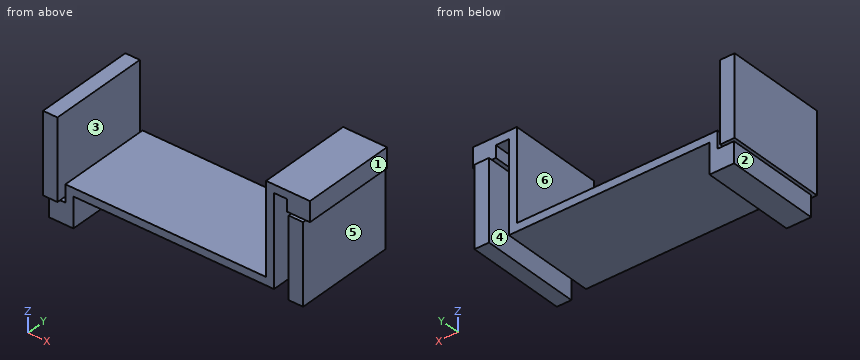
```python
from build123d import *

# Parameters (mm, degrees)
MALE_START                                 = 10.1
SKETCH_1_W                                 = 2.54
SKETCH_1_H                                 = 17.78
MALE_HOUSINGS_IN_J5_DEPTH                  = 14
FEMALE_START                               = 8.66
SKETCH_2_W                                 = 2.54
SKETCH_2_H                                 = 17.78
FEMALE_HOUSINGS_ON_THE_MODULE_HEADER_DEPTH = 14
S_BEND_START                               = 5
SKETCH_3_W                                 = 4.3
SKETCH_3_H                                 = 16.64
S_BEND_ABOVE_THE_FEMALE_HOUSINGS_DEPTH     = 3.66
SKETCH_4_W                                 = 1.4
SKETCH_4_H                                 = 16.64
S_BEND_DOWN_LEG_DEPTH                      = 6.7
RUN_START                                  = 10.3
SKETCH_5_W                                 = 36.6
SKETCH_5_H                                 = 16.64
RUN_UNDER_THE_BATTERY_DEPTH                = 1.4
DROP_START                                 = 10.3
SKETCH_6_W                                 = 1.4
SKETCH_6_H                                 = 16.64
DROP_BESIDE_THE_MODULE_EDGE_DEPTH          = 17.3
RUN_START_2                                = 26.2
SKETCH_7_W                                 = 7.7
SKETCH_7_H                                 = 16.64
RUN_UNDER_THE_MALE_HOUSINGS_DEPTH          = 1.4
LOOP_START                                 = 24.1
SKETCH_8_W                                 = 4
SKETCH_8_H                                 = 16.64
LOOP_INTO_THE_MALE_HOUSINGS_DEPTH          = 3.5


with BuildPart() as part:
    # 草圖1 → male housings in J5 (new body)
    with BuildSketch(Plane.XY.offset(MALE_START)):
        with Locations((56, 45)):
            Rectangle(SKETCH_1_W, SKETCH_1_H)
    extrude(amount=MALE_HOUSINGS_IN_J5_DEPTH)



with BuildPart() as body_2:
    # 草圖2 → female housings on the module header (new body)
    with BuildSketch(Plane.XY.offset(FEMALE_START)):
        with Locations((12.9, 45)):
            Rectangle(SKETCH_2_W, SKETCH_2_H)
    extrude(amount=FEMALE_HOUSINGS_ON_THE_MODULE_HEADER_DEPTH)

    # 草圖3 → S-bend above the female housings (add)
    with BuildSketch(Plane.XY.offset(S_BEND_START)):
        with Locations((14.35, 45)):
            Rectangle(SKETCH_3_W, SKETCH_3_H)
    extrude(amount=S_BEND_ABOVE_THE_FEMALE_HOUSINGS_DEPTH)

    # 草圖4 → S-bend down leg (add)
    with BuildSketch(Plane.XY.offset(S_BEND_START)):
        with Locations((15.8, 45)):
            Rectangle(SKETCH_4_W, SKETCH_4_H)
    extrude(amount=S_BEND_DOWN_LEG_DEPTH)

    # 草圖5 → run under the battery (add)
    with BuildSketch(Plane.XY.offset(RUN_START)):
        with Locations((33.4, 45)):
            Rectangle(SKETCH_5_W, SKETCH_5_H)
    extrude(amount=RUN_UNDER_THE_BATTERY_DEPTH)

    # 草圖6 → drop beside the module edge (add)
    with BuildSketch(Plane.XY.offset(DROP_START)):
        with Locations((51, 45)):
            Rectangle(SKETCH_6_W, SKETCH_6_H)
    extrude(amount=DROP_BESIDE_THE_MODULE_EDGE_DEPTH)

    # 草圖7 → run under the male housings (add)
    with BuildSketch(Plane.XY.offset(RUN_START_2)):
        with Locations((54.15, 45)):
            Rectangle(SKETCH_7_W, SKETCH_7_H)
    extrude(amount=RUN_UNDER_THE_MALE_HOUSINGS_DEPTH)


with BuildPart() as part_1:
    add(part.part)

    add(body_2.part)  # loop into the male housings merges body 2
    # 草圖8 → loop into the male housings (add)
    with BuildSketch(Plane.XY.offset(LOOP_START)):
        with Locations((56, 45)):
            Rectangle(SKETCH_8_W, SKETCH_8_H)
    extrude(amount=LOOP_INTO_THE_MALE_HOUSINGS_DEPTH)


solid = part_1.part
```
Read the model definition and answer for the solid it produces. Units are mm, in the model's axes. Face numbers are marked on the shaded views. A direction names the side the tool comes from. Give positions to 0.01 mm unless a question says otherwise; leave off trailing zeros. Order: outer loops, then holes, each group sorted by start corner. A loop starts at its lowest first (then second) coordinate and runs counter-clockwise, first axis right, second up.
(1) Find section B-B (y = 52.5). Give the vertices of the cut face in (x, z).
(2) Find section D-D (x = 51). Give the vertices of the cut face in (y, z), plus the area to 3 significant figures.
(3) Find section A-A (z = 19.25). Give the vertices of the cut face in (x, y).
(4) For a pull along X with two mould halves and no side action, classify the marked faces 1, 2 and 3 as released by +X, released by -X, zero draft, split by the parting line, or undercut.
(5) Given pin 1 (8 mm diameter, centred on x = 51, y = 52, fed in from -Z); pin 2 (2 mm diameter, centred on x = 13, y = 49, fed in from +Z); pin 3 (8.5 mm diameter, centred on x = 37.5, y = 42, fed in from +Z); pin 4 (0.6 mm diameter, centred on x = 55.5, y = 36.5, fed in from +Z), each flat-ended and moving along its own axis, determine where each tip first touches the part or whether it passes through.
(6) Find section C-C (z = 11). Give the vertices of the cut face in (x, y), plus the area to 3 significant figures.
(7) Straight lines are drawn through the part: L1, parallel to X at y = 41.5, z = 13; L2, parallel to X at y = 45.25, z = 11.5; L3, parallel to Z at x = 34.5, y = 45. For each, find the intervals that lie inside material, in ascending order.
(8) For the marked faces 4, 5 and 6, determine the directions among +Z, -Z, +X, -X, +Y, -Y from which every point of the face is accessible in a straight line to the end or side of a thin tool.
Result sheet:
1. outline: (11.63, 8.66) - (12.2, 8.66) - (12.2, 5) - (16.5, 5) - (16.5, 10.3) - (51.7, 10.3) - (51.7, 26.2) - (54, 26.2) - (54, 24.1) - (54.73, 24.1) - (54.73, 10.1) - (57.27, 10.1) - (57.27, 24.1) - (58, 24.1) - (58, 27.6) - (50.3, 27.6) - (50.3, 11.7) - (15.1, 11.7) - (15.1, 8.66) - (14.17, 8.66) - (14.17, 22.66) - (11.63, 22.66) - close
2. outline: (36.68, 10.3) - (53.32, 10.3) - (53.32, 27.6) - (36.68, 27.6) - close
2. area: 288 mm2
3. outline: (11.63, 36.11) - (14.17, 36.11) - (14.17, 53.89) - (11.63, 53.89) - close; (50.3, 36.68) - (51.7, 36.68) - (51.7, 53.32) - (50.3, 53.32) - close; (54.73, 36.11) - (57.27, 36.11) - (57.27, 53.89) - (54.73, 53.89) - close
4. face 1: released by +X
4. face 2: released by -X
4. face 3: undercut
5. pin 1: stops at z = 10.1
5. pin 2: stops at z = 22.66
5. pin 3: stops at z = 11.7
5. pin 4: stops at z = 27.6
6. outline: (11.63, 36.11) - (14.17, 36.11) - (14.17, 53.89) - (11.63, 53.89) - close; (15.1, 36.68) - (51.7, 36.68) - (51.7, 53.32) - (15.1, 53.32) - close; (54.73, 36.11) - (57.27, 36.11) - (57.27, 53.89) - (54.73, 53.89) - close
6. area: 699 mm2
7. L1: x = 11.63 to 14.17, 50.3 to 51.7, 54.73 to 57.27
7. L2: x = 11.63 to 14.17, 15.1 to 51.7, 54.73 to 57.27
7. L3: z = 10.3 to 11.7
8. face 4: -Z, +Y, -Y
8. face 5: -Z, +X, +Y, -Y
8. face 6: +Z, +Y, -Y
